Check sheet for the drawn part. Datum: minimum x, y, z corner. Units: mm. A direction names the side the tool comes from. Round coordinates to 2 decimals unless told otherwise and drop trailing zeros. Write each loop counter-clockwise with the first axis right and the second up, starting at its lowest first coordinate (ties: lowest second). Pieces come first, ordered by that corner, then holes. Notation, with made-up numbers: M 26.5,36.5 L 48.5,36.5 A26 ccw 48.5,61.5 Z; hole C 36,10 d5. An arc over 180 degrees is marked long. Use a Markdown table: item, result.
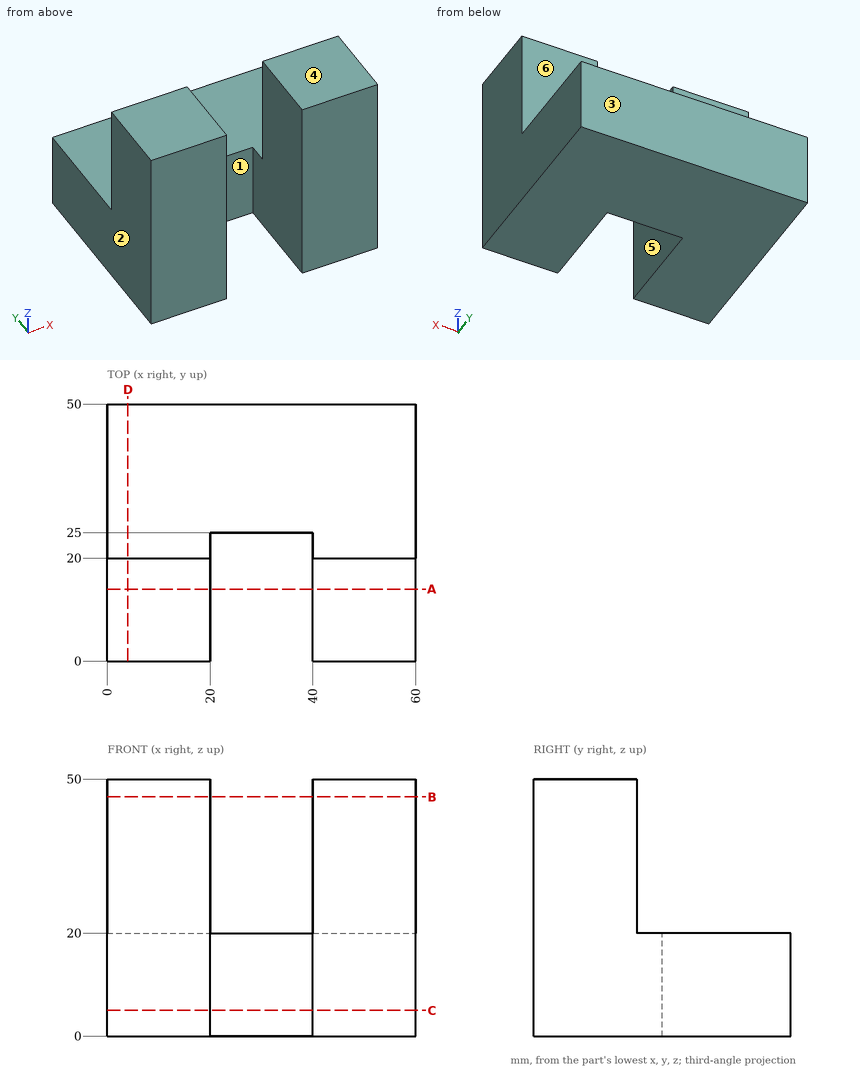
Item 1: Access from +Z, -Z, +X, -X, +Y, -Y to the whole of each face (thin tool, end or side, straight path). Record for the marked faces 4, 5 and 6.
Outcome:
| item | result |
|---|---|
| face 4 | +Z, +X, -X, +Y, -Y |
| face 5 | +Z, -Z, -Y |
| face 6 | +Z, +X, -X, +Y |
Item 2: Cross-section at B-B, the plane z = 46.5. Record the cut outline in (x, y), and give its area (3 significant figures).
Outcome:
| item | result |
|---|---|
| outline | M 0,0 L 20,0 L 20,20 L 0,20 Z; M 40,0 L 60,0 L 60,20 L 40,20 Z |
| area | 800 mm2 |
Item 3: Mould release check, pull along X, two halves, no side actions. Record for the marked faces 1, 2 and 3: +X half, -X half, draft (parallel to the pull), parting line (faces both ways), or undercut.
Outcome:
| item | result |
|---|---|
| face 1 | undercut |
| face 2 | -X half |
| face 3 | draft |
Item 4: Go/stop test with flat-tipped pins: pin 1 (1.5 mm diameter, centred on x = 22, y = 41, fed in from +Z); pin 2 (6 mm diameter, centred on x = 33, z = 12, fed in from -Y); pin 3 (6 mm diameter, centred on x = 52, z = 31, fed in from +Y). Record where each tip stops, or that it passes through.
Outcome:
| item | result |
|---|---|
| pin 1 | stops at z = 20 |
| pin 2 | stops at y = 25 |
| pin 3 | stops at y = 20 |
Item 5: Cross-section at A-A, the plane y = 14. Record the cut outline in (x, z), and give its area (3 significant figures).
Outcome:
| item | result |
|---|---|
| outline | M 0,0 L 20,0 L 20,50 L 0,50 Z; M 40,0 L 60,0 L 60,50 L 40,50 Z |
| area | 2,000 mm2 |
Item 6: Cross-section at C-C, the plane z = 5. Record the cut outline in (x, y).
Outcome:
| item | result |
|---|---|
| outline | M 0,0 L 20,0 L 20,25 L 40,25 L 40,0 L 60,0 L 60,50 L 0,50 Z |
Item 7: Material ranges on line 1 along X through (y, z) = (21, 14); line 2 along Y through (x, z) = (25.5, 15); line 3 along Y through (x, z) = (10, 37.5), recorded low to high. Write a range as from..to.
Outcome:
| item | result |
|---|---|
| line 1 | x = 0..20, 40..60 |
| line 2 | y = 25..50 |
| line 3 | y = 0..20 |
Item 8: Cross-section at D-D, the plane x = 4. Record the cut outline in (y, z).
Outcome:
| item | result |
|---|---|
| outline | M 0,0 L 50,0 L 50,20 L 20,20 L 20,50 L 0,50 Z |
